```python
from build123d import *

# Parameters (mm, degrees)
SKETCH1_W               = 30
SKETCH1_H               = 20
BOSS_EXTRUDE1_DEPTH     = 2
BOSS_EXTRUDE2_START     = -2.5
BOSS_EXTRUDE2_OUTLINE_R = 1.75
BOSS_EXTRUDE2_OUTLINE_W = 30
BOSS_EXTRUDE2_OUTLINE_H = 20
BOSS_EXTRUDE2_DEPTH     = 2.5
SKETCH5_W               = 12.800974789
SKETCH5_H               = 10
BOSS_EXTRUDE3_DEPTH     = 7.942853576
SKETCH6_R               = 1.1
CUT_EXTRUDE3_DEPTH      = 10.350916352
CUT_EXTRUDE4_DEPTH      = 10
BOSS_EXTRUDE4_START     = 4.3
SKETCH8_W               = 4.957735271
SKETCH8_H               = 12.800974789
SKETCH8_R               = 1.1
BOSS_EXTRUDE4_DEPTH     = 4.3
FILLET2_R               = 4
SKETCH9_R               = 1.7
CUT_EXTRUDE5_DEPTH      = 5


# Read off the part's stored shape, not the designer's step: Boss-Extrude2
with BuildPart() as part:
    # Sketch1 → Boss-Extrude1 (new body)
    with BuildSketch(Plane(origin=(0, 0, 0), x_dir=(0, 0, -1), z_dir=(1, 0, 0))):
        Rectangle(SKETCH1_W, SKETCH1_H)
    extrude(amount=BOSS_EXTRUDE1_DEPTH)

    # Boss-Extrude2 outline → Boss-Extrude2 (add)
    with BuildSketch(Plane(origin=(2, 0, 0), x_dir=(0, 0, -1), z_dir=(1, 0, 0)).offset(BOSS_EXTRUDE2_START)):
        with BuildLine():
            Line((-41.329654068, -16.384050837), (19.386302525, -16.711150914))
            ThreePointArc((19.386302525, -16.711150914), (24.443402602, -11.654050837), (19.386302525, -6.596950759))
            Line((19.386302525, -6.596950759), (19.386302525, 8.271904581))
            ThreePointArc((19.386302525, 8.271904581), (24.460347107, 13.345949163), (19.386302525, 18.419993745))
            Line((19.386302525, 18.419993745), (-48.501605412, 18.419993745))
            ThreePointArc((-48.501605412, 18.419993745), (-52.089496744, 16.933840495), (-53.575649994, 13.345949163))
            Line((-53.575649994, 13.345949163), (-55.414672264, 13.345949163))
            Line((-55.414672264, 13.345949163), (-55.414672264, -4.656096182))
            Line((-55.414672264, -4.656096182), (-41.753395036, -4.656096182))
            Line((-41.753395036, -4.656096182), (-41.329654068, -16.384050837))
        make_face()
        with Locations((19.386302525, -11.654050837)):
            Circle(BOSS_EXTRUDE2_OUTLINE_R, mode=Mode.SUBTRACT)
        Rectangle(BOSS_EXTRUDE2_OUTLINE_W, BOSS_EXTRUDE2_OUTLINE_H, mode=Mode.SUBTRACT)
        with Locations((19.386302525, 13.345949163)):
            Circle(BOSS_EXTRUDE2_OUTLINE_R, mode=Mode.SUBTRACT)
    extrude(amount=BOSS_EXTRUDE2_DEPTH)

    # Sketch5 → Boss-Extrude3 (add)
    with BuildSketch(Plane(origin=(2, 0, 0), x_dir=(0, 0, -1), z_dir=(1, 0, 0))):
        with Locations((-49.014184869, 0.343903818)):
            Rectangle(SKETCH5_W, SKETCH5_H)
    extrude(amount=BOSS_EXTRUDE3_DEPTH)

    # Sketch6 → Cut-Extrude3 (cut)
    with BuildSketch(Plane(origin=(4.063003727, -4.656096182, -0.641169076), x_dir=(1, 0, 0), z_dir=(0, -1, 0))):
        with Locations(Location((3.15, 48.941437628, 0), (0, 0, 270))):
            Circle(SKETCH6_R)
    extrude(amount=-CUT_EXTRUDE3_DEPTH, mode=Mode.SUBTRACT)

    # Sketch7 → Cut-Extrude4 (cut)
    with BuildSketch(Plane(origin=(2, 0, 0), x_dir=(0, 0, -1), z_dir=(1, 0, 0))):
        with BuildLine():
            Line((-34.112632424, 11.943731273), (9.404530778, 11.943731273))
            ThreePointArc((9.404530778, 11.943731273), (11.525851122, 11.065051617), (12.404530778, 8.943731273))
            Line((12.404530778, 8.943731273), (12.404530778, -6.148588701))
            ThreePointArc((12.404530778, -6.148588701), (11.525851122, -8.269909045), (9.404530778, -9.148588701))
            Line((9.404530778, -9.148588701), (-34.112632424, -9.148588701))
            ThreePointArc((-34.112632424, -9.148588701), (-36.233952768, -8.269909045), (-37.112632424, -6.148588701))
            Line((-37.112632424, -6.148588701), (-37.112632424, 8.943731273))
            ThreePointArc((-37.112632424, 8.943731273), (-36.233952768, 11.065051617), (-34.112632424, 11.943731273))
        make_face()
    extrude(amount=-CUT_EXTRUDE4_DEPTH, mode=Mode.SUBTRACT)

    # Sketch8 → Boss-Extrude4 (add)
    with BuildSketch(Plane.XZ.offset(4.656096182).offset(BOSS_EXTRUDE4_START)):
        with Locations((7.463985941, 49.014184869)):
            Rectangle(SKETCH8_W, SKETCH8_H)
        with Locations(Location((7.213003727, 48.300268552, 0), (0, 0, 270))):
            Circle(SKETCH8_R, mode=Mode.SUBTRACT)
    extrude(amount=-BOSS_EXTRUDE4_DEPTH)

    # Fillet2
    fillet2_edges = [part.edges().sort_by_distance(p)[0] for p in [
        (9.942853576, -1.806096182, 55.414672264),
        (9.942853576, -1.806096182, 42.613697475),
    ]]
    fillet(fillet2_edges, radius=FILLET2_R)

    # Sketch9 → Cut-Extrude5 (cut)
    with BuildSketch(Plane(origin=(2, 0, 0), x_dir=(0, 0, -1), z_dir=(1, 0, 0))):
        with Locations((-47.255689875, 9.377983735)):
            Circle(SKETCH9_R)
    extrude(amount=-CUT_EXTRUDE5_DEPTH, mode=Mode.SUBTRACT)


solid = part.part
```
Geometry: final body of the model. Coordinates: model frame, mm. A direction names the side the tool comes from. Round coordinates to 2 decimals unless told otherwise and drop trailing zeros. Loops run counter-clockwise (first coordinate to the right, second up) from the corner with the lowest first, then second, coordinate; pieces in that order, holes last. Notation, with made-up numbers: (64.5, 5) -> (92.5, 5) arc R35 ccw to (92.5, 44) -> close; hole circle Ø7 at (37.5, -19.75). An arc over 180 degrees is marked (long way). Use one line per item in the form item = value. Start each with the question number.
1) Draft query along Y for faces 1 (the flat face through (1, -9.149, 12)), 2 (the flat face through (6, 5.344, 49)), 3 (the flat face through (2, 13, 16)). Return one class per face: released by +Y, released by -Y, zero draft, split by the parting line, or undercut.
2) Section B-B on x = 1.25. Output: boundary loops of the cut face in (y, z).
3) First-contact query: P1, Ø0.6, axis at x = 0, z = -14, coming from the -Y side; P2, Ø0.8, axis at x = 1, z = 3.5, coming from the -Y side; P3, Ø3, axis at x = 4.5, y = -1.5, coming from the -Z side; P4, Ø5.5, axis at y = -11.65, z = -19.39, coming from the -X side. Flat tips, straight axial feed; report the tip coordinate or a pass-through.
4) Section A-A on z = 16.5. Output: boundary loops of the cut face in (x, y).
5) Section C-C on z = 0. Output: boundary loops of the cut face in (x, y), then the cut area to 3 significant figures.
6) Section D-D on y = 16. Output: boundary loops of the cut face in (x, z).
7) Access query for faces 4 (the flat face through (1, 11.944, 13)), 5 (the flat face through (1, 13.346, 54)), 6 (the flat face through (1, 1, -19.386)). Directions: +Z, -Z, +X, -X, +Y, -Y. A direction counts if a zero-diameter tool reaches every point of the face in a straight line with its end or side. Return the directions, or none.
8) Line query: L1, parallel to Z at x = 1.25, y = 8; L2, parallel to Y at x = 7, z = 52; L3, parallel to X at y = 10.5, z = -14.5. Output: solid intervals per line, ascending.
Response:
q1.face_1 = undercut
q1.face_2 = released by +Y
q1.face_3 = zero draft
q2.outline = (-16.71, -19.39) arc R5.06 ccw to (-6.6, -19.39) -> (8.27, -19.39) arc R5.07 ccw to (18.42, -19.39) -> (18.42, 48.5) arc R5.07 ccw to (13.35, 53.58) -> (13.35, 55.41) -> (-4.66, 55.41) -> (-4.66, 41.75) -> (-16.38, 41.33) -> close; hole circle Ø3.5 at (-11.65, -19.39); hole (-9.15, -9.4) arc R3 ccw to (-6.15, -12.4) -> (8.94, -12.4) arc R3 ccw to (11.94, -9.4) -> (11.94, 34.11) arc R3 ccw to (8.94, 37.11) -> (-6.15, 37.11) arc R3 ccw to (-9.15, 34.11) -> close; hole circle Ø3.4 at (9.38, 47.26); hole circle Ø3.5 at (13.35, -19.39)
q3.P1 = -16.68
q3.P2 = -16.59
q3.P3 = 42.61
q3.P4 = -0.5
q4.outline = (-0.5, -16.52) -> (2, -16.52) -> (2, -9.15) -> (-0.5, -9.15) -> close; (-0.5, 11.94) -> (2, 11.94) -> (2, 18.42) -> (-0.5, 18.42) -> close
q5.outline = (-0.5, -16.61) -> (2, -16.61) -> (2, -9.15) -> (0, -9.15) -> (0, -10) -> (-0.5, -10) -> close; (-0.5, 11.94) -> (2, 11.94) -> (2, 18.42) -> (-0.5, 18.42) -> close
q5.area = 34.4 mm^2
q6.outline = (-0.5, -23.71) -> (2, -23.71) -> (2, 52.83) -> (-0.5, 52.83) -> close
q7.face_4 = +X, -X
q7.face_5 = +Z, +X, -X, +Y
q7.face_6 = -Z, +X, -X
q8.L1 = -19.39 to -12.4, 37.11 to 46.26, 48.25 to 55.41
q8.L2 = -8.96 to 5.34
q8.L3 = -0.5 to 2
